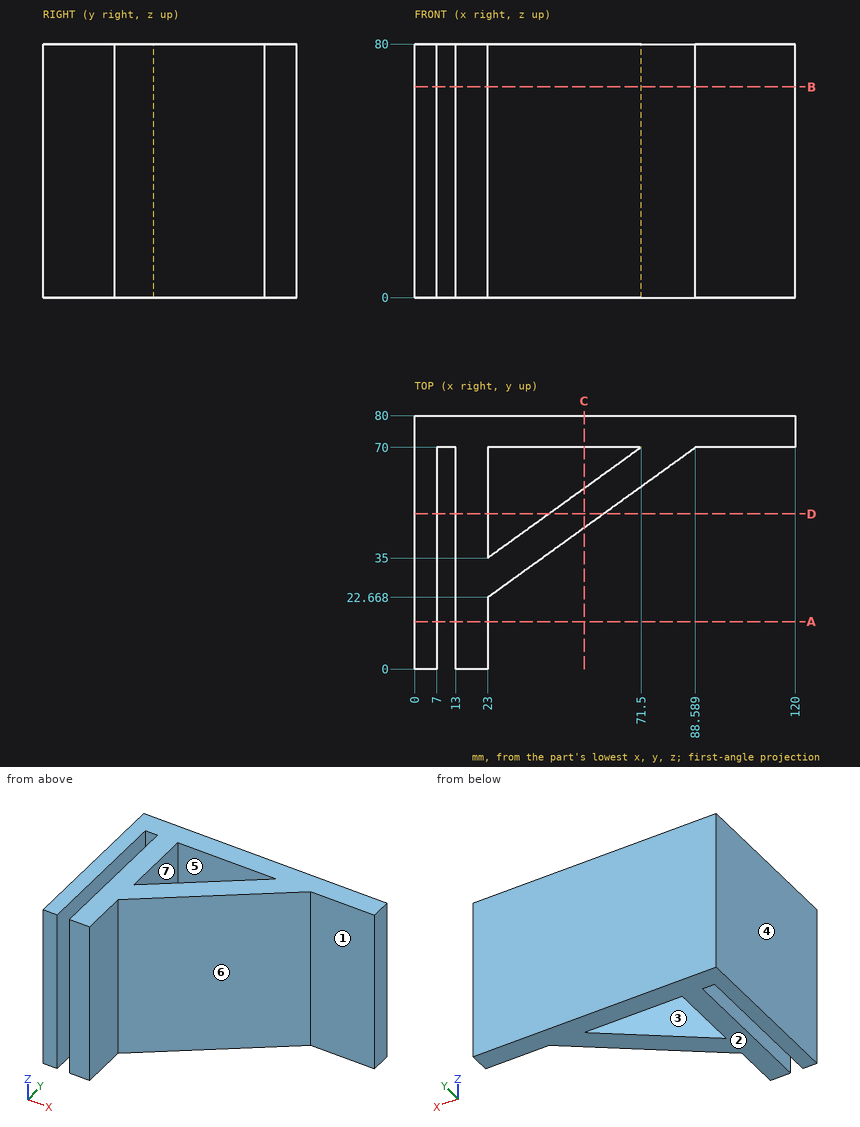
Here's the drawing with two shaded views (mm, measured from the low corner). I have some questions. A direction names the side the tool comes from. Give positions to 0.01 mm unless a question says otherwise; leave off trailing zeros. Write each loop counter-clockwise with the first axis right and the second up, starting at its lowest first coordinate (ties: lowest second). Pieces come first, ordered by that corner, then holes. Notation, with made-up numbers: (-12, 38) -> (21, 38) arc R19 ccw to (21, 74) -> close; hole circle Ø8 at (43, -12). An arc over 180 degrees is marked (long way). One line per item, written item: value.
Q1. Imagine slicing it at D-D on y = 49. Please give me the cut outline in (x, z).
Results found:
outline: (0, 0) -> (7, 0) -> (7, 80) -> (0, 80) -> close; (13, 0) -> (23, 0) -> (23, 80) -> (13, 80) -> close; (42.4, 0) -> (59.49, 0) -> (59.49, 80) -> (42.4, 80) -> close
Q2. For P1, Ø14.5, axis at x = 43.5, z = 51.5, coming from the -Y side; P2, Ø2, axis at y = 22.5, z = 43.5, coming from the +X side; P3, Ø7, axis at y = 10.5, z = 39, coming from the +X side, each with a flat end and sliding along its axis, tell me the tip position at first contact or that it passes through.
Results found:
P1: stops at y = 32.23
P2: stops at x = 24.15
P3: stops at x = 23
Q3. Which directions (+Z, -Z, +X, -X, +Y, -Y) give clear straight access to the entire face, cutting with the end or side of a thin tool? Please do the marked faces 1, 2 and 3.
Results found:
face 1: +Z, -Z, +X, -Y
face 2: -Z, +X, -X, +Y, -Y
face 3: +Z, -Z
Q4. We'd pull the mould along Y, two halves only. Please class the marked faces 4, 5, 6 and 7: +Y half, -Y half, draft (parallel to the pull), parting line (faces both ways), or undercut.
Results found:
face 4: draft
face 5: undercut
face 6: -Y half
face 7: undercut
Q5. Please list where these lines run through material, in increasing order: line 1 (X direction, y = 19.5, z = 45); line 2 (X direction, y = 55.5, z = 54) (1 decimal); line 3 (X direction, y = 50.5, z = 58.5) (1 decimal). Write a range as [from, to].
Results found:
line 1: x = [0, 7], [13, 23]
line 2: x = [0, 7], [13, 23], [51.4, 68.5]
line 3: x = [0, 7], [13, 23], [44.5, 61.6]
Q6. Imagine slicing it at A-A on y = 15. Please give me the cut outline in (x, z), and give its area (3 significant figures).
Results found:
outline: (0, 0) -> (7, 0) -> (7, 80) -> (0, 80) -> close; (13, 0) -> (23, 0) -> (23, 80) -> (13, 80) -> close
area: 1,360 mm^2
Q7. Imagine slicing it at B-B on z = 66.5. Please give me the cut outline in (x, y), and give its area (3 significant figures).
Results found:
outline: (0, 0) -> (7, 0) -> (7, 70) -> (13, 70) -> (13, 0) -> (23, 0) -> (23, 22.67) -> (88.59, 70) -> (120, 70) -> (120, 80) -> (0, 80) -> close; hole (23, 35) -> (71.5, 70) -> (23, 70) -> close
area: 3,090 mm^2
Q8. Imagine slicing it at C-C on x = 53.5. Please give me the cut outline in (y, z).
Results found:
outline: (44.68, 0) -> (57.01, 0) -> (57.01, 80) -> (44.68, 80) -> close; (70, 0) -> (80, 0) -> (80, 80) -> (70, 80) -> close
